Drawing for the job (mm, zero at the part's lowest x, y, z). Give positions to 0.01 mm unless a question says otherwise; leave off trailing zeros. Write each loop counter-clockwise with the first axis right and the second up, starting at its lowest first coordinate (ties: lowest second). Pieces come first, ordered by that corner, then holes. Notation, with made-up numbers: M 53.25,-14 L 74.25,-14 A13 cw 74.25,9 Z; hole C -13,83.25 d3. An arc over 180 degrees is marked long. Answer as a JSON object with one key per item and string values. Group by question number.
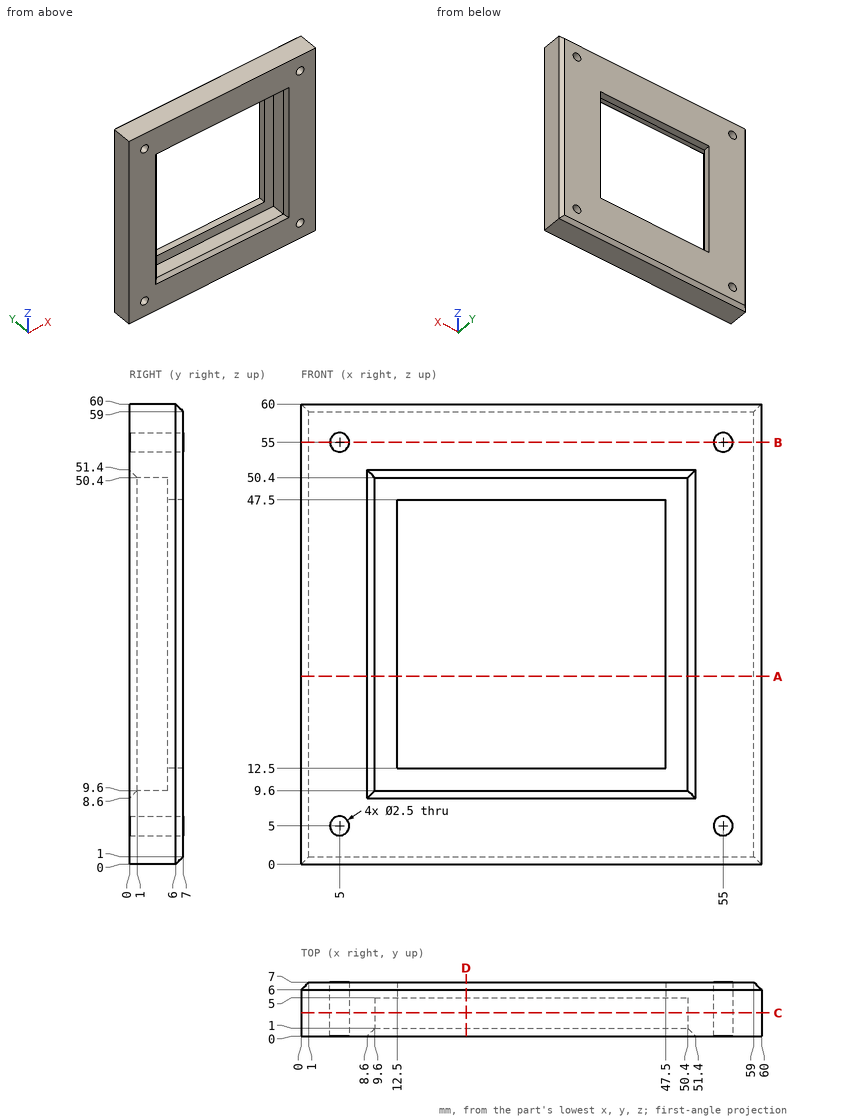
Q1. Wall check: L1, parallel to Z at x = 55, y = 3; L2, parallel to Z at x = 13, y = 5.25. Give the ranges that are in metal, low to high.
Q2. Slice it at D-D, the plane x = 21.5. Write the cut outline in (y, z).
Q3. Drop flat-ended pins along their axis: P1, Ø2, axis at x = 5, z = 55, coming from the -Y side; P2, Ø10, axis at x = 27.5, z = 15.5, coming from the -Y side. Give the stop position or say it passes through.
Q4. Slice it at A-A, the plane z = 24.5. Write the cut outline in (x, y), then the cut area to 3 significant figures.
Q5. Slice it at C-C, the plane y = 3. Write the cut outline in (x, z).
Q6. Slice it at B-B, the plane z = 55. Write the cut outline in (x, y), then the cut area to 3 significant figures.
Solved:
{
 "1": {"L1": "z = 0 to 3.75, 6.25 to 53.75, 56.25 to 60", "L2": "z = 0 to 12.5, 47.5 to 60"},
 "2": {"outline": "M 0,0 L 6,0 L 7,1 L 7,12.5 L 5,12.5 L 5,9.6 L 1,9.6 L 0,8.6 Z; M 0,51.4 L 1,50.4 L 5,50.4 L 5,47.5 L 7,47.5 L 7,59 L 6,60 L 0,60 Z"},
 "3": {"P1": "passes through", "P2": "stops at y = 5"},
 "4": {"outline": "M 0,0 L 8.6,0 L 9.6,1 L 9.6,5 L 12.5,5 L 12.5,7 L 1,7 L 0,6 Z; M 47.5,5 L 50.4,5 L 50.4,1 L 51.4,0 L 60,0 L 60,6 L 59,7 L 47.5,7 Z", "area": "144 mm²"},
 "5": {"outline": "M 0,0 L 60,0 L 60,60 L 0,60 Z; hole C 5,5 d2.5; hole C 5,55 d2.5; hole M 9.6,9.6 L 50.4,9.6 L 50.4,50.4 L 9.6,50.4 Z; hole C 55,5 d2.5; hole C 55,55 d2.5"},
 "6": {"outline": "M 0,0 L 3.75,0 L 3.75,7 L 1,7 L 0,6 Z; M 6.25,0 L 53.75,0 L 53.75,7 L 6.25,7 Z; M 56.25,0 L 60,0 L 60,6 L 59,7 L 56.25,7 Z", "area": "384 mm²"}
}
